Design review of the part built by this model. Coordinates are the model's own, in mm. A direction names the side the tool comes from. Coordinates: 2 decimals unless noted, no trailing zeros. Loops run counter-clockwise (first coordinate to the right, second up) from the corner with the lowest first, then second, coordinate; pieces in that order, holes last. Notation, with made-up numbers: (4.5, 1) -> (49.5, 1) arc R31 cw to (49.5, 26) -> close; hole circle Ø3 at (-22.5, -35). An arc over 180 degrees is marked (long way). Use a Markdown table: item, result. Add a question column.
Q1. Take a section at B-B on y = 16. Write out the cut boundary in (x, z).
Q2. Take a section at C-C on y = 11.25. Write out the cut boundary in (x, z), plus the area to 3 significant figures.
Q3. Take a section at D-D on x = 4.5. Count the separate pieces of the cut face and the enclosed holes in it, plus the area to 3 significant figures.
Q4. For faces 4 (the face through (3, 0, 3)), 5 (the face through (5.535, 4.536, 0.325)), list the 3-axis set-ups (+Z, -Z, +X, -X, +Y, -Y) from which the entire face can be reached by the end or side of a thin tool; tool diameter is ignored.
Q5. For probe 1 along Y at (x, z) = (4.5, 0); probe 2 along X at (y, z) = (8, 0); probe 3 along Y at (x, z) = (5.5, 1.25), list the stretches that pass through material, from the lowest coordinate up.
Q6. Draft analysis for pull direction X (two halves, no side actions). For faces 1 (the face through (-1.73, 10.86, 7.81)), 2 (the face through (3, 11, 0)), 3 (the face through (5.53, 17.01, 1.11)), state which applies: pulls with the +X half, pulls with the -X half, needs draft (parallel to the pull), parting line crosses it, or undercut.
Q7. Clearance check with flat-ended pins moving along their axes: pin 1 Ø6 at (x, z) = (-1.5, 0.5) entering from -Y; pin 2 Ø3 at (y, z) = (8.5, 3.5) entering from +X; pin 3 Ø2 at (x, y) = (1.5, 14.5) entering from +Z; pin 4 Ø2 at (y, z) = (13.5, -4) entering from +X. State where each tip first meets the part, or that it passes through.
Q8. Take a section at A-A on z = 0. Write out the cut boundary in (x, y), plus the area to 3 significant figures.
from build123d import *

# Parameters (mm, degrees)
SKETCH1_R           = 8
BOSS_EXTRUDE1_DEPTH = 22
CUT_EXTRUDE3_DEPTH  = 12
CUT_EXTRUDE4_DEPTH  = 10
CHAMFER1_SIZE       = 1
CUT_EXTRUDE5_REACH  = 18
SKETCH4_R           = 1.5


with BuildPart() as part:
    # Sketch1 → Boss-Extrude1 (new body)
    with BuildSketch(Plane(origin=(0, 0, 0), x_dir=(1, 0, 0), z_dir=(0, 1, 0))):
        Circle(SKETCH1_R)
    extrude(amount=BOSS_EXTRUDE1_DEPTH)

    # Sketch3 → Cut-Extrude3 (cut)
    with BuildSketch(Plane.XZ):
        with BuildLine():
            Line((3, 2.645751311), (3, -2.645751311))
            ThreePointArc((3, -2.645751311), (-4, 0), (3, 2.645751311))
        make_face()
    extrude(amount=-CUT_EXTRUDE3_DEPTH, mode=Mode.SUBTRACT)

    # Sketch2 → Cut-Extrude4 (cut)
    with BuildSketch(Plane(origin=(0, 22, 0), x_dir=(1, 0, 0), z_dir=(0, 1, 0))):
        with BuildLine():
            Line((3, 2.645751311), (3, -2.645751311))
            ThreePointArc((3, -2.645751311), (1.645751311, -3.645751311), (0, -4))
            ThreePointArc((0, -4), (-4, 0), (0, 4))
            ThreePointArc((0, 4), (1.645751311, 3.645751311), (3, 2.645751311))
        make_face()
    extrude(amount=-CUT_EXTRUDE4_DEPTH, mode=Mode.SUBTRACT)

    # Chamfer1
    chamfer1_edges = [part.edges().sort_by_distance(p)[0] for p in [
        (-8, 0, 0),
        (-8, 22, 0),
    ]]
    chamfer(chamfer1_edges, length=CHAMFER1_SIZE)

    # Sketch4 → Cut-Extrude5 (cut, up to next)
    with BuildSketch(Plane(origin=(8, 0, 0), x_dir=(0, 0, -1), z_dir=(1, 0, 0)), mode=Mode.PRIVATE) as cut_extrude5_sk1:
        with Locations((0, 16)):
            Circle(SKETCH4_R)
    cut_extrude5_tool1 = extrude(cut_extrude5_sk1.sketch, amount=-CUT_EXTRUDE5_REACH, mode=Mode.PRIVATE) & part.part
    add(cut_extrude5_tool1.solids().sort_by_distance((8, 16, 0))[0], mode=Mode.SUBTRACT)
    # Sketch4 → Cut-Extrude5 (cut, up to next)
    with BuildSketch(Plane(origin=(8, 0, 0), x_dir=(0, 0, -1), z_dir=(1, 0, 0)), mode=Mode.PRIVATE) as cut_extrude5_sk2:
        with Locations((0, 6)):
            Circle(SKETCH4_R)
    cut_extrude5_tool2 = extrude(cut_extrude5_sk2.sketch, amount=-CUT_EXTRUDE5_REACH, mode=Mode.PRIVATE) & part.part
    add(cut_extrude5_tool2.solids().sort_by_distance((8, 6, 0))[0], mode=Mode.SUBTRACT)


solid = part.part
Answer list:
| question | item | result |
|---|---|---|
| 1 | outline | (3, -2.65) arc R4 cw (long way) to (3, 2.65) -> (3, 1.5) -> (7.86, 1.5) arc R8 ccw (long way) to (7.86, -1.5) -> (3, -1.5) -> close |
| 2 | outline | circle Ø16 at (0, 0); hole (3, -2.65) -> (3, 2.65) arc R4 ccw (long way) to start |
| 2 | area | 154 mm² |
| 3 | separate pieces | 1 |
| 3 | enclosed holes | 2 |
| 3 | area | 274 mm² |
| 4 | face 4 | +Z, -Z, +X, -X, -Y |
| 4 | face 5 | +X |
| 5 | probe 1 | 0 to 4.5, 7.5 to 14.5, 17.5 to 22 |
| 5 | probe 2 | -8 to -4, 3 to 8 |
| 5 | probe 3 | 0 to 5.17, 6.83 to 15.17, 16.83 to 22 |
| 6 | face 1 | parting line crosses it |
| 6 | face 2 | undercut |
| 6 | face 3 | needs draft |
| 7 | pin 1 | y = 0 |
| 7 | pin 2 | x = 7.75 |
| 7 | pin 3 | z = 7.98 |
| 7 | pin 4 | x = 7.42 |
| 8 | outline | (-8, 1) -> (-7, 0) -> (-4, 0) -> (-4, 22) -> (-7, 22) -> (-8, 21) -> close; (3, 0) -> (7, 0) -> (8, 1) -> (8, 4.5) -> (3, 4.5) -> close; (3, 7.5) -> (8, 7.5) -> (8, 14.5) -> (3, 14.5) -> close; (3, 17.5) -> (8, 17.5) -> (8, 21) -> (7, 22) -> (3, 22) -> close |
| 8 | area | 166 mm² |
